Source: CAD feature listing. Evaluate the final solid. Frame: model axes, mm. Round coordinates to 2 decimals unless told otherwise and drop trailing zeros. Order: outer loops, then holes, each group sorted by start corner. A loop starts at its lowest first (then second) coordinate and runs counter-clockwise, first axis right, second up. Notation, with made-up numbers: (-27.75, -15.75) - (-7.75, -15.75) arc R32 ccw to (-7.75, 23.25) - close; hole circle Ø7 at (-17, 60.5). An arc over 180 degrees is marked (long way). Return JSON: item names as keys, results as strings. Group by question number.
1) Section B-B, the plane y = -5.15. Return loops of the section in (x, z), plus the area to 3 significant figures.
2) Section A-A, the plane x = 0. Return loops of the section in (y, z), plus the area to 3 significant figures.
3) Ray query, line 1 (Z direction, x = -4, y = -3.2); line 2 (Z direction, x = 1.75, y = -5.45); line 3 (X direction, y = -5.4, z = -4.75). Return the intervals inside material, ascending. Write a range as from..to.
4) Contact query for flat-ended pins moving along their axis: P1, Ø3, axis at y = -3.5, z = 2.5, coming from the +X side; P2, Ø2, axis at y = -2.5, z = -5, coming from the +X side; P3, Ø1.5, axis at y = -2.5, z = 3, coming from the +X side. Output: stop coordinate, or through.
```python
from build123d import *

# Parameters (mm, degrees)
F1_DEPTH = 6
F2_R     = 6
F3_DEPTH = 25
F4_R     = 0.5


with BuildPart() as f1:
    # F0 (on Front) → F1 (new body)
    with BuildSketch(Plane.XZ):
        Polygon((5.1961524227, 9), (-5.1961524227, 9), (-10.3923048454, 0), (-5.1961524227, -9), (5.1961524227, -9), (10.3923048454, 0), align=None)
    extrude(amount=F1_DEPTH)

    # F2 (on face) → F3 (cut)
    with BuildSketch(Plane.XZ.offset(6)):
        Circle(F2_R)
    extrude(amount=-F3_DEPTH, mode=Mode.SUBTRACT)

    # F4
    f4_edges = [f1.edges().sort_by_distance(p)[0] for p in [
        (7.794229, -6, 4.5),
        (7.794229, -6, -4.5),
        (0, -6, 9),
        (0, -6, -9),
        (-7.794229, -6, 4.5),
        (-7.794229, -6, -4.5),
        (-6, -6, 0),
        (-6, 0, 0),
    ]]
    fillet(f4_edges, radius=F4_R)


solid = f1.part
```
Geometry check:
{
 "1": {"outline": "(-10.39, 0) - (-5.2, -9) - (5.2, -9) - (10.39, 0) - (5.2, 9) - (-5.2, 9) - close; hole circle Ø12 at (0, 0)", "area": "167 mm2"},
 "2": {"outline": "(-6, -8.5) arc R0.5 ccw to (-5.5, -9) - (0, -9) - (0, -6.5) arc R0.5 ccw to (-0.5, -6) - (-5.5, -6) arc R0.5 ccw to (-6, -6.5) - close; (-6, 6.5) arc R0.5 ccw to (-5.5, 6) - (-0.5, 6) arc R0.5 ccw to (0, 6.5) - (0, 9) - (-5.5, 9) arc R0.5 ccw to (-6, 8.5) - close", "area": "35.7 mm2"},
 "3": {"line 1": "-9..-4.47, 4.47..9", "line 2": "-9..-5.74, 5.74..9", "line 3": "-7.65..-3.67, 3.67..7.65"},
 "4": {"P1": "x = 9.81", "P2": "x = 8.08", "P3": "x = 9.09"}
}
